```python
from build123d import *

# Parameters (mm, degrees)
SCHIZZO1_R                   = 4.5
SCHIZZO1_R_2                 = 2
ESTRUSIONE_ESTRUSIONE1_DEPTH = 5


with BuildPart() as part:
    # Schizzo1 → Estrusione-Estrusione1 (new body)
    with BuildSketch(Plane.XY):
        with BuildLine():
            Line((0, -15), (50, -15))
            ThreePointArc((50, -15), (57.434856863, -6.513641332), (48.044417196, -0.259440913))
            ThreePointArc((48.044417196, -0.259440913), (28.031173765, -0.132787617), (10.933286622, 10.269529864))
            ThreePointArc((10.933286622, 10.269529864), (-13.766679846, 5.956385315), (0, -15))
        make_face()
        Circle(SCHIZZO1_R, mode=Mode.SUBTRACT)
        with Locations((50, -7.5)):
            Circle(SCHIZZO1_R_2, mode=Mode.SUBTRACT)
    extrude(amount=ESTRUSIONE_ESTRUSIONE1_DEPTH)


solid = part.part
```
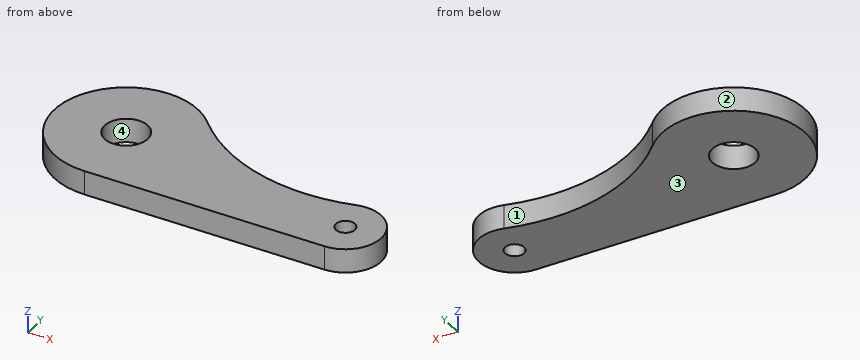
The listing builds one solid part. Answer for the finished solid, in the listing's coordinates (mm). Face numbers are marked on the shaded views. Give positions to 0.01 mm unless a question says otherwise; leave off trailing zeros. Order: outer loops, then holes, each group sorted by start corner. A loop starts at its lowest first (then second) coordinate and runs counter-clockwise, first axis right, second up. Notation, with made-up numbers: (-18, 16.5) -> (36, 16.5) arc R25 ccw to (36, 45.5) -> close; hole circle Ø2 at (-11.75, 11.25). An arc over 180 degrees is marked (long way). Answer as CSV lines item,"result". Start each with the question number.
Q1. A cutting plane is placed at C-C (y = 2.75). Determine the outline of the cut face in (x, z), then the cut area to 3 significant figures.
Q2. A cutting plane is placed at B-B (z = 0.95). Determine the outline of the cut face in (x, y), then the cut area to 3 significant figures.
Q3. A cutting plane is placed at D-D (x = 36). Determine the outline of the cut face in (y, z), then the cut area to 3 significant figures.
Q4. Given pin 1 (1 mm diameter, centred on x = -3, z = 4, fed in from +Y); pin 2 (1 mm diameter, centred on x = -7, z = 0.5, fed in from +Y); pin 3 (1 mm diameter, centred on x = 31, z = 2.5, fed in from +Y), each flat-ended and moving along its own axis, determine where each tip first touches the part or whether it passes through.
Q5. Determine the mould class of the marked faces 1, 2, 3 and 4 for opening direction X: pulls with the +X half, pulls with the -X half, needs draft (parallel to the pull), parting line crosses it, or undercut.
Q6. A cutting plane is placed at A-A (y = -3). Determine the outline of the cut face in (x, z), then the cut area to 3 significant figures.
Q7. Find the intervals of material crossed by L1, parallel to Y at x = 50, z = 2.65; L2, parallel to Y at x = 0, z = 1.8; L3, parallel to X at y = 3, z = 0.95, in increasing order.
Results found:
1,outline,"(-14.75, 0) -> (-3.56, 0) -> (-3.56, 5) -> (-14.75, 5) -> close; (3.56, 0) -> (20.82, 0) -> (20.82, 5) -> (3.56, 5) -> close"
1,area,"142 mm2"
2,outline,"(0, -15) -> (50, -15) arc R7.5 ccw (long way) to (48.04, -0.26) arc R37.5 cw to (10.93, 10.27) arc R15 ccw (long way) to start; hole circle Ø9 at (0, 0); hole circle Ø4 at (50, -7.5)"
2,area,"1,310 mm2"
3,outline,"(-15, 0) -> (-1.49, 0) -> (-1.49, 5) -> (-15, 5) -> close"
3,area,"67.6 mm2"
4,pin 1,"y = 14.79"
4,pin 2,"y = 13.52"
4,pin 3,"y = -0.74"
5,face 1,"undercut"
5,face 2,"parting line crosses it"
5,face 3,"needs draft"
5,face 4,"undercut"
6,outline,"(-14.7, 0) -> (-3.35, 0) -> (-3.35, 5) -> (-14.7, 5) -> close; (3.35, 0) -> (56, 0) -> (56, 5) -> (3.35, 5) -> close"
6,area,"320 mm2"
7,L1,"-15 to -9.5, -5.5 to 0"
7,L2,"-15 to -4.5, 4.5 to 15"
7,L3,"-14.7 to -3.35, 3.35 to 20.35"
